Autodesk Inventor part; units mm, degrees
ref_plane "YZ Plane" through (0, 0, 0) normal (1, 0, 0) x (0, 1, 0)
ref_plane "XZ Plane" through (0, 0, 0) normal (0, 1, 0) x (-1, 0, 0)
ref_plane "XY Plane" through (0, 0, 0) normal (0, 0, 1) x (1, 0, 0)
sketch "Sketch_1" plane through (0, 0, 0) normal (0, 1, 0) x (-1, 0, 0)
  arc A0 (20, 17) -> (17, 20) centre (17, 17) ccw
  line L0 (17, 20) -> (-17, 20)
  arc A1 (-17, 20) -> (-20, 17) centre (-17, 17) ccw
  line L1 (-20, 17) -> (-20, -17)
  arc A2 (-20, -17) -> (-17, -20) centre (-17, -17) ccw
  line L2 (-17, -20) -> (17, -20)
  arc A3 (17, -20) -> (20, -17) centre (17, -17) ccw
  line L3 (20, -17) -> (20, 17)
extrude "Extrusion1" add sketch "Sketch_1" along normal blind 52
sketch "Sketch_2" plane through (0, 0, 0) normal (1, 0, 0) x (0, 1, 0)
  line L0 (12, 20) -> (52, -20)
  line L1 (52, -20) -> (52, 20)
  line L2 (52, 20) -> (12, 20)
extrude "Extrusion2" cut sketch "Sketch_2" along normal mid plane 40
sketch "Sketch_13" plane through (0, 0, 0) normal (1, 0, 0) x (0, 1, 0)
  line L0 (13.4142, 21.4142) -> (12, 20)
  line L1 (12, 20) -> (17.3033, 14.6967)
  line L2 (17.3033, 14.6967) -> (18.7175, 16.1109)
  line L3 (18.7175, 16.1109) -> (13.4142, 21.4142)
extrude "Extrusion3" add sketch "Sketch_13" along normal mid plane 7.7
sketch "Sketch_14" plane through (0, 0, 0) normal (1, 0, 0) x (0, 1, 0)
  line L0 (47.7574, -12.9289) -> (46.3431, -14.3431)
  line L1 (46.3431, -14.3431) -> (52, -20)
  line L2 (52, -20) -> (53.4142, -18.5858)
  line L3 (53.4142, -18.5858) -> (47.7574, -12.9289)
extrude "Extrusion4" add sketch "Sketch_14" along normal mid plane 7.7
sketch "Sketch_3" plane through (0, 15.5, 0) normal (0, 1, 0) x (1, 0, 0)
  line L0 (-16.8, -23.5) -> (-10.8, -23.5)
  line L1 (-10.8, -23.5) -> (-10.8, 16.5)
  line L2 (-10.8, 16.5) -> (-16.8, 16.5)
  line L3 (-16.8, 16.5) -> (-16.8, -23.5)
extrude "Extrusion5" cut sketch "Sketch_3" along normal blind 40
sketch "Sketch_4" plane through (0, 15.5, 0) normal (0, 1, 0) x (1, 0, 0)
  line L0 (10.8, -23.5) -> (16.8, -23.5)
  line L1 (16.8, -23.5) -> (16.8, 16.5)
  line L2 (16.8, 16.5) -> (10.8, 16.5)
  line L3 (10.8, 16.5) -> (10.8, -23.5)
extrude "Extrusion6" cut sketch "Sketch_4" along normal blind 40
sketch "Sketch_5" plane through (0, 10, 0) normal (0, 1, 0) x (1, 0, 0)
  line L0 (-7.5, 0.5) -> (-7.5, -7.5)
  line L1 (-7.5, -7.5) -> (7.5, -7.5)
  line L2 (7.5, -7.5) -> (7.5, 0.5)
  arc A0 (7.5, 0.5) -> (-7.5, 0.5) centre (0, 0.5) ccw
extrude "Extrusion7" cut sketch "Sketch_5" along normal blind 40
sketch "Sketch_6" plane through (0, 0, 0) normal (1, 0, 0) x (0, 1, 0)
  line L0 (50, 20) -> (22.5, 20)
  line L1 (22.5, 20) -> (10, 7.5)
  line L2 (10, 7.5) -> (50, 7.5)
  line L3 (50, 7.5) -> (50, 20)
extrude "Extrusion8" cut sketch "Sketch_6" along normal mid plane 15
sketch "Sketch9" plane through (0, 10, 0) normal (0, 1, 0) x (1, 0, 0)
  point P0 (0, 0)
hole "Hole1" at (0, 10, 0) direction (0, -1, 0) diameter 9 depth 10
sketch "Sketch_8" plane through (0, 0, 14.3841) normal (0, -0.7071, 0.7071) x (1, 0, 0)
  line L0 (-4.5, -2.7) -> (-4.5, -3.5714)
  line L1 (-4.5, -3.5714) -> (4.5, -3.5714)
  line L2 (4.5, -3.5714) -> (4.5, -2.7)
  arc A0 (4.5, -2.7) -> (1.8, 0) centre (1.8, -2.7) ccw
  line L3 (1.8, 0) -> (-1.8, 0)
  arc A1 (-1.8, 0) -> (-4.5, -2.7) centre (-1.8, -2.7) ccw
extrude "Extrusion9" cut sketch "Sketch_8" against normal blind 20
sketch "Sketch_9" plane through (0, 0, 0) normal (1, 0, 0) x (0, 1, 0)
  line L0 (0, 9.67) -> (0, 0)
  line L1 (0, 0) -> (10, 0)
  line L2 (10, 0) -> (10, 4.3841)
  line L3 (10, 4.3841) -> (4.7141, 9.67)
  line L4 (4.7141, 9.67) -> (0, 9.67)
extrude "Extrusion10" cut sketch "Sketch_9" along normal mid plane 3
sketch "Sketch_10" plane through (0, 0, 0) normal (1, 0, 0) x (0, 1, 0)
  line L0 (0.7957, 9.77) -> (0, 9.77)
  line L1 (0, 9.77) -> (0, 0)
  line L2 (0, 0) -> (10, 0)
  line L3 (10, 0) -> (10, 0.5657)
  line L4 (10, 0.5657) -> (0.7957, 9.77)
extrude "Extrusion11" cut sketch "Sketch_10" along normal mid plane 9
sketch "Sketch_11" plane through (0, 0, 0) normal (1, 0, 0) x (0, 1, 0)
  line L0 (27.9584, -24.2426) -> (42.1005, -10.1005)
  line L1 (42.1005, -10.1005) -> (45.2825, -13.2825)
  line L2 (45.2825, -13.2825) -> (31.1403, -27.4246)
  line L3 (31.1403, -27.4246) -> (27.9584, -24.2426)
  line L4 (27.9584, -24.2426) -> (42.1005, -10.1005)
revolve "Revolution1" cut sketch "Sketch_11" angle 360 about axis through (0, 27.9584, -24.2426) along (0, -0.7071, -0.7071)
sketch "Sketch_15" plane through (0, 0, 0) normal (1, 0, 0) x (0, 1, 0)
  line L0 (0, 20) -> (-2, 18)
  line L1 (-2, 18) -> (-0.9393, 16.9393)
  line L2 (-0.9393, 16.9393) -> (1.0607, 18.9393)
  line L3 (1.0607, 18.9393) -> (0, 20)
extrude "Extrusion12" add sketch "Sketch_15" along normal mid plane 8
sketch "Sketch_16" plane through (0, 0, 0) normal (1, 0, 0) x (0, 1, 0)
  line L0 (0, -15.8787) -> (-2, -17.8787)
  line L1 (-2, -17.8787) -> (-0.9393, -18.9393)
  line L2 (-0.9393, -18.9393) -> (1.0607, -16.9393)
  line L3 (1.0607, -16.9393) -> (0, -15.8787)
extrude "Extrusion13" add sketch "Sketch_16" along normal mid plane 8
sketch "Sketch_12" plane through (0, 28.4645, -3.5355) normal (0, 0.7071, 0.7071) x (1, 0, 0)
  arc A0 (-7.5, 14.3) -> (7.5, 14.3) centre (0, 14.3) ccw
  line L0 (7.5, 14.3) -> (7.5, 23.3)
  line L1 (7.5, 23.3) -> (-7.5, 23.3)
  line L2 (-7.5, 23.3) -> (-7.5, 14.3)
extrude "Extrusion14" cut sketch "Sketch_12" against normal blind 40
sketch "Sketch_17" plane through (9, 0, 0) normal (1, 0, 0) x (0, 0, -1)
  line L0 (-15, 12.5) -> (-15, 0)
  line L1 (-15, 0) -> (15, 0)
  line L2 (15, 0) -> (2.5, 12.5)
  line L3 (2.5, 12.5) -> (-15, 12.5)
extrude "Extrusion15" cut sketch "Sketch_17" along normal blind 7
sketch "Sketch_18" plane through (-9, 0, 0) normal (1, 0, 0) x (0, 0, -1)
  line L0 (-15, 12.5) -> (-15, 0)
  line L1 (-15, 0) -> (15, 0)
  line L2 (15, 0) -> (2.5, 12.5)
  line L3 (2.5, 12.5) -> (-15, 12.5)
extrude "Extrusion16" cut sketch "Sketch_18" against normal blind 7
properties part number "14118"
Geometry: final body of the model. Coordinates: model frame, mm. A direction names the side the tool comes from. Coordinates: 2 decimals unless noted, no trailing zeros. Order: outer loops, then holes, each group sorted by start corner. A loop starts at its lowest first (then second) coordinate and runs counter-clockwise, first axis right, second up. Notation, with made-up numbers: (55.5, -2.5) - (76.5, -2.5) arc R19 cw to (76.5, 16.5) - close; hole circle Ø10 at (79.25, 25). An arc over 180 degrees is marked (long way). Write each question's results on one line, items separated by ' | '.
1) Pull-direction query (X, two-part tool) for faces 5 (the flat face through (-1.772, 41.775, -16.843)), 6 (the flat face through (20, 19, -4)), 7 (the flat face through (-0.05, 16.08, 18.75)); classes: pulls with the +X half, pulls with the -X half, needs draft (parallel to the pull), parting line crosses it, or undercut.
Results list:
face 5: undercut | face 6: pulls with the +X half | face 7: needs draft
2) Line query: line 1 (X direction, y = 5, z = 4); line 2 (X direction, y = 38.5, z = -13.5); line 3 (Y direction, x = -12, z = 10.5). Output: solid intervals per line, ascending. Write a range as from..to.
Results list:
line 1: -20..-16, -9..-4.5, 4.5..9, 16..20 | line 2: -20..-16.8, -10.8..-4.5, 4.5..10.8, 16.8..20 | line 3: 12.5..15.5
3) Pin query (flat end, axial travel): pin 1 (8 mm diameter, centred on y = 27.5, z = 13, fed in from -X); pin 2 (3.5 mm diameter, centred on x = 8, y = 4, fed in from +Z); pin 3 (1.8 mm diameter, centred on x = 15, y = 38.5, fed in from +Z); pin 4 (5 mm diameter, centred on x = 6, z = -10.5, fed in from +Y). Return the tip coordinate at first contact, or that it passes through.
Results list:
pin 1: through | pin 2: z = 20 | pin 3: z = -16.5 | pin 4: y = 45
4) Section B-B, the plane y = 16.5. Return loops of the section in (x, z).
Results list:
outline: (-20, -17) arc R3 ccw to (-17, -20) - (17, -20) arc R3 ccw to (20, -17) - (20, 15.5) - (16.8, 15.5) - (16.8, -16.5) - (10.8, -16.5) - (10.8, 15.5) - (3.85, 15.5) - (3.85, 18.33) - (-3.85, 18.33) - (-3.85, 15.5) - (-10.8, 15.5) - (-10.8, -16.5) - (-16.8, -16.5) - (-16.8, 15.5) - (-20, 15.5) - close; hole (-7.5, -0.5) arc R7.5 ccw to (7.5, -0.5) - (7.5, 14) - (-7.5, 14) - close
5) Section A-A, the plane x = 0. State how many separate pieces and enclosed holes the cut face has, plus the area to 3 significant figures.
Results list:
separate pieces: 3 | enclosed holes: 0 | area: 601 mm^2
6) Set-up query: faces 1 (the flat face through (-0.1, 14.4, 11.9)), 2 (the flat face through (16.8, 24, -7)), 3 (the flat face through (0.025, 4.93, 9.454)), 4 (the flat face through (-4, -1, 18)). Return all of +Z, -Z, +X, -X, +Y, -Y with unobstructed straight access to the full face (end or side cutting, diameter ignored); none if empty.
Results list:
face 1: +Y | face 2: +Z, +Y | face 3: -Y | face 4: +Z, -Z, -X, -Y
7) Section C-C, the plane x = 14. Return loops of the section in (y, z), plus the area to 3 significant figures.
Results list:
outline: (0, -20) - (52, -20) - (48.5, -16.5) - (15.5, -16.5) - (15.5, 16.5) - (12, 20) - (0, 20) - (0, 15) - (12.5, 15) - (12.5, -2.5) - (0, -15) - close | area: 439 mm^2
